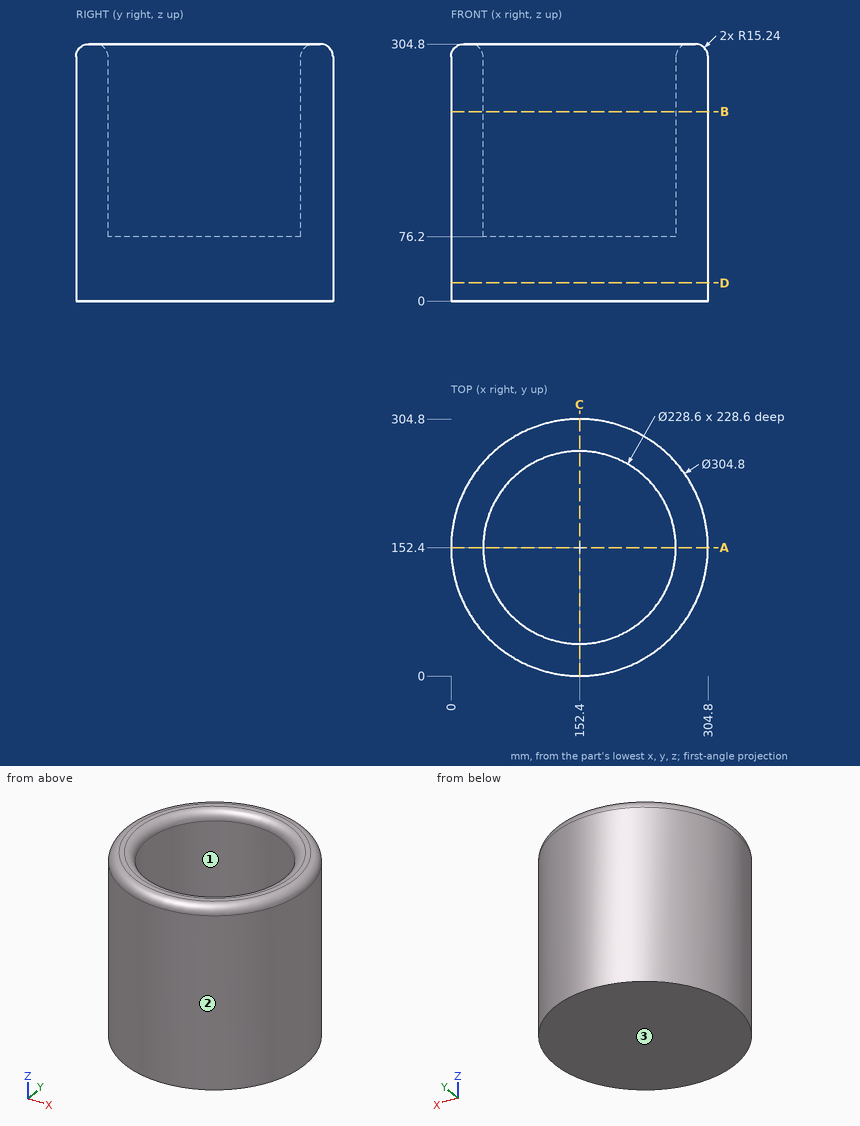
For this review, use the dimensioned drawing (mm, ordinates from the lowest corner) and the shaded views. Round coordinates to 2 decimals unless told otherwise and drop trailing zeros. Write each loop counter-clockwise with the first axis right and the second up, starting at its lowest first coordinate (ties: lowest second). Pieces come first, ordered by that corner, then holes. Notation, with made-up numbers: M -39,61.5 L -4,61.5 A13 ccw -4,69.5 Z; hole C 70.25,-7.5 d1. An arc over 180 degrees is marked long. Answer as CSV lines item,"result". Start each with the question number.
Q1. Wall thickness on line 1 along X through (y, z) = (152, 187); line 2 along Z through (x, y) = (53.5, 248): over which ranges is each line inside the solid? List them lowest first.
Q2. Consider section D-D, the plane z = 21.5. Give the boundary of the cut face in (x, y).
Q3. Consider section A-A, the plane y = 152.4. Give the boundary of the cut face in (x, z), then the cut area to 3 significant figures.
Q4. Clearance check with flat-ended pins moving along their axes: P1, Ø2, axis at y = 35.5, z = 139.5, coming from the -X side; P2, Ø1.5, axis at x = 180, z = 68.5, coming from the +Y side; P3, Ø12, axis at x = 77.5, y = 111.5, coming from the +Z side. State where each tip first meets the part, or that it passes through.
Q5. The part is to be moulded in two halves that separate along Y. For the marked faces 1, 2 and 3, say which applies: +Y half, -Y half, draft (parallel to the pull), parting line (faces both ways), or undercut.
Q6. Consider section B-B, the plane z = 224.5. Give the boundary of the cut face in (x, y).
Result set:
1,line 1,"x = 0 to 38.1, 266.7 to 304.8"
1,line 2,"z = 0 to 304.79"
2,outline,"C 152.4,152.4 d304.8"
3,outline,"M 0,0 L 304.8,0 L 304.8,289.56 A15.24 ccw 289.56,304.8 L 281.94,304.8 A15.24 ccw 266.7,289.56 L 266.7,76.2 L 38.1,76.2 L 38.1,289.56 A15.24 ccw 22.86,304.8 L 15.24,304.8 A15.24 ccw 0,289.56 Z"
3,area,"40,400 mm²"
4,P1,"stops at x = 53.44"
4,P2,"stops at y = 302.42"
4,P3,"stops at z = 76.2"
5,face 1,"undercut"
5,face 2,"parting line"
5,face 3,"draft"
6,outline,"C 152.4,152.4 d304.8; hole C 152.4,152.4 d228.6"
